```python
from build123d import *

# Parameters (mm, degrees)
F0_W     = 47
F0_H     = 24
F1_DEPTH = 15
F3_DEPTH = 13
F4_R     = 1
F5_DEPTH = 10


with BuildPart() as f1:
    # F0 (on Top) → F1 (new body)
    with BuildSketch(Plane.XY):
        Rectangle(F0_W, F0_H)
    extrude(amount=F1_DEPTH)

    # F2 (on face) → F3 (cut)
    with BuildSketch(Plane.XY.offset(15)):
        with BuildLine():
            Line((21.5, 10), (18, 10))
            Line((18, 10), (18, 7.5))
            ThreePointArc((18, 7.5), (15, 4.5), (12, 7.5))
            Line((12, 7.5), (12, 10))
            Line((12, 10), (-21.5, 10))
            Line((-21.5, 10), (-21.5, -10))
            Line((-21.5, -10), (-18, -10))
            Line((-18, -10), (-18, -7.5))
            ThreePointArc((-18, -7.5), (-15, -4.5), (-12, -7.5))
            Line((-12, -7.5), (-12, -10))
            Line((-12, -10), (21.5, -10))
            Line((21.5, -10), (21.5, 10))
        make_face()
    extrude(amount=-F3_DEPTH, mode=Mode.SUBTRACT)

    # F4 (on face) → F5 (cut)
    with BuildSketch(Plane.XY.offset(15)):
        with Locations((15, 7.5)):
            Circle(F4_R)
        with Locations((-15, -7.5)):
            Circle(F4_R)
    extrude(amount=-F5_DEPTH, mode=Mode.SUBTRACT)


solid = f1.part
```
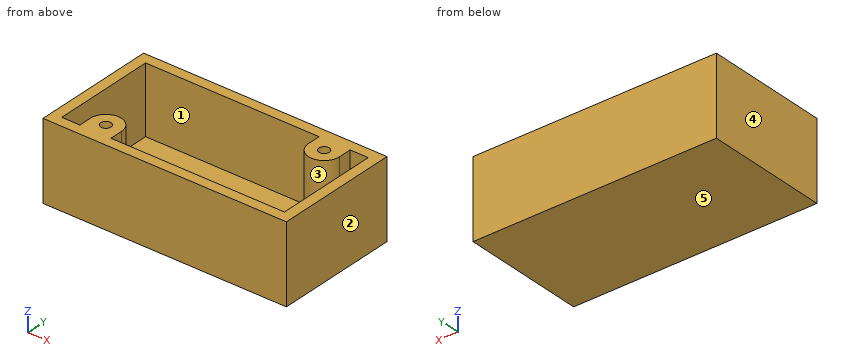
Work out the finished part from the listing and answer in its coordinate system (mm). Face numbers are marked on the shaded views. A direction names the side the tool comes from. Give positions to 0.01 mm unless a question says otherwise; leave off trailing zeros. Loops run counter-clockwise (first coordinate to the right, second up) from the corner with the lowest first, then second, coordinate; pieces in that order, holes last. Notation, with made-up numbers: (41.5, 59.5) -> (94.5, 59.5) arc R32 cw to (94.5, 90.5) -> close; hole circle Ø4 at (82.5, 58). An arc over 180 degrees is marked (long way). Use CSV: the item, a comma, the result in double quotes.
1. The part is cut by section C-C (y = -2.75). Write down the section's boundary in (x, z), then the cut area to 3 significant figures.
Found:
outline,"(-23.5, 0) -> (23.5, 0) -> (23.5, 15) -> (21.5, 15) -> (21.5, 2) -> (-21.5, 2) -> (-21.5, 15) -> (-23.5, 15) -> close"
area,"146 mm^2"
2. Straight lines are drawn through the part: line 1 (X direction, y = 9.5, z = 5.5); line 2 (Y direction, x = -15, z = 10); line 3 (Y direction, x = 15, z = 12). For each, find the intervals that lie inside material, in ascending order.
Found:
line 1,"-23.5 to -21.5, 12 to 18, 21.5 to 23.5"
line 2,"-12 to -8.5, -6.5 to -4.5, 10 to 12"
line 3,"-12 to -10, 4.5 to 6.5, 8.5 to 12"
3. The mould has two halves that part along X. Classify the marked faces 3, 4 and 5: +X half, -X half, draft (parallel to the pull), parting line (faces both ways), or undercut.
Found:
face 3,"undercut"
face 4,"-X half"
face 5,"draft"
4. Flat-ended cylindrical pins translate along their axes: pin 1 Ø1 at (x, y) = (-0.5, 5) entering from +Z; pin 2 Ø1.6 at (x, y) = (15, 7.5) entering from +Z. Find the tip coordinate at first contact, or state that the pin passes through.
Found:
pin 1,"z = 2"
pin 2,"z = 5"
5. The part is cut by section A-A (z = 10.75). Write down the section's boundary in (x, y).
Found:
outline,"(-23.5, -12) -> (23.5, -12) -> (23.5, 12) -> (-23.5, 12) -> close; hole (-21.5, -10) -> (-18, -10) -> (-18, -7.5) arc R3 cw to (-12, -7.5) -> (-12, -10) -> (21.5, -10) -> (21.5, 10) -> (18, 10) -> (18, 7.5) arc R3 cw to (12, 7.5) -> (12, 10) -> (-21.5, 10) -> close; hole circle Ø2 at (-15, -7.5); hole circle Ø2 at (15, 7.5)"
6. The part is cut by section D-D (z = 3.25). Write down the section's boundary in (x, y).
Found:
outline,"(-23.5, -12) -> (23.5, -12) -> (23.5, 12) -> (-23.5, 12) -> close; hole (-21.5, -10) -> (-18, -10) -> (-18, -7.5) arc R3 cw to (-12, -7.5) -> (-12, -10) -> (21.5, -10) -> (21.5, 10) -> (18, 10) -> (18, 7.5) arc R3 cw to (12, 7.5) -> (12, 10) -> (-21.5, 10) -> close"
7. A tool of negligible diameter and unlimited length cuts with its end or side. For the marked faces 1 and 2, from which of +Z, -Z, +X, -X, +Y, -Y can it reach the whole face along a straight path? Write none if from no direction.
Found:
face 1,"+Z"
face 2,"+Z, -Z, +X, +Y, -Y"
8. The part is cut by section B-B (x = -15). Write down the section's boundary in (y, z), then the cut area to 4 significant figures.
Found:
outline,"(-12, 0) -> (12, 0) -> (12, 15) -> (10, 15) -> (10, 2) -> (-4.5, 2) -> (-4.5, 15) -> (-6.5, 15) -> (-6.5, 5) -> (-8.5, 5) -> (-8.5, 15) -> (-12, 15) -> close"
area,"151.5 mm^2"
